Build history of the part. All positions in model axes, mm. A direction names the side the tool comes from. Give positions to 0.01 mm unless a question says otherwise; leave off trailing zeros. Order: outer loops, then holes, each group sorted by start corner. A loop starts at its lowest first (then second) coordinate and runs counter-clockwise, first axis right, second up. Notation, with made-up numbers: (-18, 85) -> (28, 85) arc R24 cw to (28, 120) -> close; hole circle Ø1 at (41.5, 16.25). An arc over 180 degrees is marked (long way). Use a Markdown table: item, result. Add a question column.
```python
from build123d import *

# Parameters (mm, degrees)
SKETCH_1_W               = 3.76
SKETCH_1_H               = 11.54
SKETCH_1_W_2             = 1.83
SKETCH_1_W_3             = 14.6
SKETCH_1_H_2             = 2.72
SKETCH_1_H_3             = 6.9
EXTRUDE_1_DEPTH          = 1
SKETCH_1_3_W             = 3.76
SKETCH_1_3_H             = 11.54
SKETCH_1_3_W_2           = 1.83
SKETCH_1_3_W_3           = 14.6
SKETCH_1_3_H_2           = 2.72
EXTRUDE_2_DEPTH          = 10
EXTRUDE_3_DEPTH          = 14.6
CUT_EXTRUDE_1_DEPTH      = 14.6
CUT_EXTRUDE_2_DEPTH      = 14.6
CUT_EXTRUDE_3_DEPTH      = 14.6
PATTERN_CIRCULAR_1_COUNT = 2
SKETCH_7_W               = 20.64829466
SKETCH_7_H               = 2.860597992
CUT_EXTRUDE_4_DEPTH      = 38.6
SKETCH_8_W               = 54.18
SKETCH_8_H               = 19.048575036
SKETCH_8_W_2             = 7
SKETCH_8_H_2             = 4.5
SKETCH_8_R               = 1.6
EXTRUDE_4_DEPTH          = 1.5
SKETCH_9_W               = 54.18
SKETCH_9_H               = 1.8
EXTRUDE_5_DEPTH          = 7
SKETCH_10_R              = 1.65
CUT_EXTRUDE_5_DEPTH      = 5
EXTRUDE_START            = 2
SKETCH_8_3_W             = 7
SKETCH_8_3_H             = 4.5
SKETCH_8_3_R             = 1.6
EXTRUDE_6_DEPTH          = 2
SKETCH_11_W              = 54.18
SKETCH_11_H              = 6.653379434
CUT_EXTRUDE_6_DEPTH      = 5


with BuildPart() as part:
    # Sketch 1 → Extrude 1 (new body)
    # profile 1 of 6: a face of its own
    with BuildSketch(Plane(origin=(0, 0, 0), x_dir=(1, 0, 0), z_dir=(0, 1, 0))):
        Polygon((-7.603, 6.17), (-7.603, -6.17), (1.387, -6.17), (1.387, -3.45), (1.387, 3.45), (1.387, 6.17), align=None)
        with Locations((-4.723, 0)):
            Rectangle(SKETCH_1_W, SKETCH_1_H, mode=Mode.SUBTRACT)
        with Locations((-0.728, 0)):
            Rectangle(SKETCH_1_W_2, SKETCH_1_H, mode=Mode.SUBTRACT)
    # profile 2 of 6: a face of its own
    with BuildSketch(Plane(origin=(0, 0, 0), x_dir=(1, 0, 0), z_dir=(0, 1, 0))):
        with Locations((8.687, -4.81)):
            Rectangle(SKETCH_1_W_3, SKETCH_1_H_2)
    # profile 3 of 6: a face of its own
    with BuildSketch(Plane(origin=(0, 0, 0), x_dir=(1, 0, 0), z_dir=(0, 1, 0))):
        with Locations((8.687, 0)):
            Rectangle(SKETCH_1_W_3, SKETCH_1_H_3)
    # profile 4 of 6: a face of its own
    with BuildSketch(Plane(origin=(0, 0, 0), x_dir=(1, 0, 0), z_dir=(0, 1, 0))):
        with Locations((8.687, 4.81)):
            Rectangle(SKETCH_1_W_3, SKETCH_1_H_2)
    # profile 5 of 6: a face of its own
    with BuildSketch(Plane(origin=(0, 0, 0), x_dir=(1, 0, 0), z_dir=(0, 1, 0))):
        with Locations((-4.723, 0)):
            Rectangle(SKETCH_1_W, SKETCH_1_H)
    # profile 6 of 6: a face of its own
    with BuildSketch(Plane(origin=(0, 0, 0), x_dir=(1, 0, 0), z_dir=(0, 1, 0))):
        with Locations((-0.728, 0)):
            Rectangle(SKETCH_1_W_2, SKETCH_1_H)
    extrude(amount=-EXTRUDE_1_DEPTH)

    # Sketch 1_3 → Extrude 2 (add)
    with BuildSketch(Plane(origin=(0, 0, 0), x_dir=(1, 0, 0), z_dir=(0, 1, 0))):
        with Locations((-4.723, 0)):
            Rectangle(SKETCH_1_3_W, SKETCH_1_3_H)
        with Locations((-0.728, 0)):
            Rectangle(SKETCH_1_3_W_2, SKETCH_1_3_H)
        with Locations((8.687, -4.81)):
            Rectangle(SKETCH_1_3_W_3, SKETCH_1_3_H_2)
        with Locations((8.687, 4.81)):
            Rectangle(SKETCH_1_3_W_3, SKETCH_1_3_H_2)
    extrude(amount=EXTRUDE_2_DEPTH)

    # Sketch 4 → Extrude 3 (add)
    with BuildSketch(Plane(origin=(15.987, 0, 0), x_dir=(0, 0, -1), z_dir=(1, 0, 0))):
        Polygon((6.17, 10), (7.707580576, 7.443577481), (7.707580576, 1.805314446), (6.17, -1), align=None)
        Polygon((-7.707580576, 1.805314446), (-6.17, -1), (-6.17, 10), (-7.707580576, 7.443577481), align=None)
    extrude(amount=-EXTRUDE_3_DEPTH)

    # Sketch 3 → Cut-Extrude 1 (cut)
    with BuildSketch(Plane(origin=(15.987, 0, 0), x_dir=(0, 0, -1), z_dir=(1, 0, 0))):
        with BuildLine():
            Line((3.45, 0), (3.743222721, 0))
            add(Edge.make_bspline(
                [(3.743222721, 0), (3.911611309, 0.15963804), (4.29393083, 0.539845441), (4.994683036, 1.333496486), (5.723480991, 2.402845903), (6.251271172, 3.695549278), (6.429364414, 5), (6.251271172, 6.304450722), (5.723480991, 7.597154097), (4.994683036, 8.666503514), (4.253106755, 9.506390689), (3.815688064, 9.935054209), (3.597380816, 10.136172737)],
                knots=[0.014828564, 0.014828564, 0.014828564, 0.014828564, 0.0625, 0.125, 0.25, 0.375, 0.5, 0.625, 0.75, 0.875, 0.9375, 0.998871937, 0.998871937, 0.998871937, 0.998871937], degree=3))
            Line((3.597380816, 10.136172737), (3.45, 10))
            Line((3.45, 10), (3.45, 0))
        make_face()
        with BuildLine():
            Line((-3.45, 0), (-3.743222721, 0))
            add(Edge.make_bspline(
                [(-3.743222721, 0), (-3.781981306, 0.035623699), (-3.849464206, 0.098316559), (-4.072000203, 0.30899054), (-4.461726475, 0.698324492), (-5.152564834, 1.48074741), (-5.881362789, 2.550096827), (-6.40915297, 3.842800202), (-6.587246212, 5.147250924), (-6.40915297, 6.451701646), (-5.881362789, 7.744405021), (-5.152564834, 8.813754438), (-4.461708764, 9.596197415), (-4.071967827, 9.985543512), (-3.84942965, 10.196217487), (-3.781968617, 10.258889811), (-3.743222721, 10.294501848)],
                knots=[0, 0, 0, 0, 0.010893382, 0.018155637, 0.0625, 0.125, 0.25, 0.375, 0.5, 0.625, 0.75, 0.875, 0.9375, 0.981850307, 0.989110184, 1, 1, 1, 1], degree=3))
            Line((-3.743222721, 10.294501848), (-3.45, 10))
            Line((-3.45, 10), (-3.45, 0))
        make_face()
    extrude(amount=-CUT_EXTRUDE_1_DEPTH, mode=Mode.SUBTRACT)

    # Sketch 5 → Cut-Extrude 2 (cut)
    with BuildSketch(Plane(origin=(0.187, 0, 0), x_dir=(0, 0, -1), z_dir=(1, 0, 0))):
        Polygon((1.17, 2.8), (-3.569711506, 4.901860767), (-5.77, 4.901860767), (-5.77, 10), (5.77, 10), (5.77, 0.3), (1.17, 0.3), align=None)
    extrude(amount=-CUT_EXTRUDE_2_DEPTH, mode=Mode.SUBTRACT)

    # Sketch 6 → Cut-Extrude 3 (cut)
    with BuildSketch(Plane(origin=(-2.843, 0, 0), x_dir=(0, 0, -1), z_dir=(1, 0, 0))):
        Polygon((1.17, 5.538552109), (1.17, 1.8), (-3.795527251, 1.8), (-5.77, 1.8), (-5.77, 5.538552109), align=None)
    extrude(amount=-CUT_EXTRUDE_3_DEPTH, mode=Mode.SUBTRACT)


with BuildPart() as pattern_circular_1_1:
    # Pattern Circular 1: pattern copy
    add(part.part.rotate(Axis((19.487, -1.5500525, 0), (0, 1, 0)), 1 * 360 / PATTERN_CIRCULAR_1_COUNT))


with BuildPart() as cut_extrude_4_tool:
    # Sketch 7 → Cut-Extrude 4 (new body)
    with BuildSketch(Plane.ZY.offset(-1.387)):
        with Locations((-0.112362095, 10.62761907)):
            Rectangle(SKETCH_7_W, SKETCH_7_H)
    extrude(amount=-CUT_EXTRUDE_4_DEPTH)


with BuildPart() as part_1:
    add(part.part)

    # Cut-Extrude 4: cut by cut_extrude_4_tool
    add(cut_extrude_4_tool.part, mode=Mode.SUBTRACT)



with BuildPart() as pattern_circular_1_1_1:
    add(pattern_circular_1_1.part)

    # Cut-Extrude 4: cut by cut_extrude_4_tool
    add(cut_extrude_4_tool.part, mode=Mode.SUBTRACT)


with BuildPart() as part_2:
    add(part_1.part)

    add(pattern_circular_1_1_1.part)  # Extrude 4 merges Pattern Circular 1_1
    # Sketch 8 → Extrude 4 (add)
    # profile 1 of 3: a face of its own
    with BuildSketch(Plane(origin=(0, 0, 0), x_dir=(1, 0, 0), z_dir=(0, 1, 0))):
        with Locations((19.487, 0)):
            Rectangle(SKETCH_8_W, SKETCH_8_H)
    # profile 2 of 3: a face of its own
    with BuildSketch(Plane(origin=(0, 0, 0), x_dir=(1, 0, 0), z_dir=(0, 1, 0))):
        with Locations((19.487, -11.774287518)):
            Rectangle(SKETCH_8_W_2, SKETCH_8_H_2)
        with Locations(Location((19.487, -11.774287518, 0), (0, 0, 270))):
            Circle(SKETCH_8_R, mode=Mode.SUBTRACT)
    # profile 3 of 3: a face of its own
    with BuildSketch(Plane(origin=(0, 0, 0), x_dir=(1, 0, 0), z_dir=(0, 1, 0))):
        with Locations((19.487, 11.774287518)):
            Rectangle(SKETCH_8_W_2, SKETCH_8_H_2)
        with Locations(Location((19.487, 11.774287518, 0), (0, 0, 270))):
            Circle(SKETCH_8_R, mode=Mode.SUBTRACT)
    extrude(amount=-EXTRUDE_4_DEPTH)

    # Sketch 9 → Extrude 5 (add)
    with BuildSketch(Plane(origin=(0, 0, 0), x_dir=(1, 0, 0), z_dir=(0, 1, 0))):
        with Locations((19.487, 8.624287518)):
            Rectangle(SKETCH_9_W, SKETCH_9_H)
    extrude(amount=EXTRUDE_5_DEPTH)

    # Sketch 10 → Cut-Extrude 5 (cut)
    with BuildSketch(Plane.XY.offset(-7.724287518)):
        with Locations((-4.603, 2.5)):
            Circle(SKETCH_10_R)
        with Locations((43.577, 2.5)):
            Circle(SKETCH_10_R)
    extrude(amount=-CUT_EXTRUDE_5_DEPTH, mode=Mode.SUBTRACT)

    # Sketch 8_3 → Extrude 6 (add)
    # profile 1 of 2: a face of its own
    with BuildSketch(Plane(origin=(0, 0, 0), x_dir=(1, 0, 0), z_dir=(0, 1, 0)).offset(EXTRUDE_START)):
        with Locations((19.487, -11.774287518)):
            Rectangle(SKETCH_8_3_W, SKETCH_8_3_H)
        with Locations(Location((19.487, -11.774287518, 0), (0, 0, 270))):
            Circle(SKETCH_8_3_R, mode=Mode.SUBTRACT)
    # profile 2 of 2: a face of its own
    with BuildSketch(Plane(origin=(0, 0, 0), x_dir=(1, 0, 0), z_dir=(0, 1, 0)).offset(EXTRUDE_START)):
        with Locations((19.487, 11.774287518)):
            Rectangle(SKETCH_8_3_W, SKETCH_8_3_H)
        with Locations(Location((19.487, 11.774287518, 0), (0, 0, 270))):
            Circle(SKETCH_8_3_R, mode=Mode.SUBTRACT)
    extrude(amount=-EXTRUDE_6_DEPTH)

    # Sketch 11 → Cut-Extrude 6 (cut, symmetric)
    with BuildSketch(Plane(origin=(0, 0, 0), x_dir=(1, 0, 0), z_dir=(0, 1, 0))):
        with Locations((19.487, -11.034270293)):
            Rectangle(SKETCH_11_W, SKETCH_11_H)
    extrude(amount=CUT_EXTRUDE_6_DEPTH, both=True, mode=Mode.SUBTRACT)


solid = part_2.part
```
(1) Tool access for faces 1 (the face through (-5, 1, 5.77)), 2 (the face through (40, 4.902, -5)), 3 (the face through (40, 2, 1.17)): list every direction of +Z, -Z, +X, -X, +Y, -Y with a clear straight run to the whole face (end or side of a thin tool).
(2) Band-saw the part on B-B on y = 3.5. State how many separate pieces and enclosed holes the cut face has, plus the area to 3 significant figures.
(3) Band-saw the part on A-A on z = -12.25. Give the cut face in (x, y).
(4) Mould opens along X. For faces 4 (the face through (22.987, 4, -7)), 5 (the face through (8.789, 8.333, -7.173)), 6 (the face through (-6.603, 1, 1)) say: released by +X, released by -X, zero draft, split by the parting line, or undercut.
(5) Wall check: probe 1 along X at (y, z) = (2.5, -6.75); probe 2 along Y at (x, z) = (-4.5, 6.75); probe 3 along X at (y, z) = (0, -10.5). Give the ranges that are in metal, low to high.
(6) Pin check, flat tips, straight feed: pin 1 Ø2 at (x, y) = (43.5, 0.5) entering from -Z; pin 2 Ø2 at (x, y) = (43.577, 2.5) entering from +Z; pin 3 Ø0.5 at (y, z) = (0.5, -2) entering from +X. Stop position of each tip, or through.
Response:
| question | item | result |
|---|---|---|
| 1 | face 1 | +Z, -X, +Y |
| 1 | face 2 | +Z, +X, -X, +Y |
| 1 | face 3 | +Z, +X, +Y |
| 2 | separate pieces | 9 |
| 2 | enclosed holes | 0 |
| 2 | area | 196 mm² |
| 3 | outline | (15.99, -1.5) -> (17.96, -1.5) -> (17.96, 2) -> (15.99, 2) -> close; (21.01, -1.5) -> (22.99, -1.5) -> (22.99, 2) -> (21.01, 2) -> close |
| 4 | face 4 | undercut |
| 4 | face 5 | zero draft |
| 4 | face 6 | released by -X |
| 5 | probe 1 | x = 1.39 to 15.99, 22.99 to 37.59 |
| 5 | probe 2 | y = -1.5 to 0 |
| 5 | probe 3 | x = 15.99 to 18.52, 20.45 to 22.99 |
| 6 | pin 1 | stops at z = -9.52 |
| 6 | pin 2 | stops at z = 1.17 |
| 6 | pin 3 | stops at x = 45.58 |
